Could you check a few things on this model? Use its own coordinates, in mm. Round coordinates to 2 decimals unless told otherwise and drop trailing zeros. Write each loop counter-clockwise with the first axis right and the second up, starting at its lowest first coordinate (ties: lowest second). Pieces come first, ordered by that corner, then holes. Notation, with made-up numbers: (84, -26.5) -> (91, -26.5) arc R13 ccw to (91, -22.5) -> close; hole circle Ø6 at (57.25, 32.5). An arc over 180 degrees is marked (long way). One line per question, with ' | ' between items. Start each with the question number.
1. Thinking about a two-plate mould opening in X: for faces 1 (the cylindrical face through (-98, 2, -99)), 2 (the cylindrical face through (7.509, 1.726, 23.846)), 3 (the cylindrical face through (98, 2, -99)), which applies, released by +X, released by -X, zero draft, split by the parting line, or undercut?
2. Imagine slicing it at B-B, the plane x = 12. List the corners of the cut face in (y, z) for me, and give its area (3 significant figures).
3. Imagine slicing it at A-A, the plane y = 1.8. State how many separate pieces and enclosed holes the cut face has, and give its area (3 significant figures).
4. If I drill on line 1 along X through (y, z) = (2.05, -94); line 2 along Z through (x, y) = (94, 1.75); line 3 along X through (y, z) = (1.9, 90), over which ranges is the centre line in solid material (lowest first)? Write a range as [from, to].
from build123d import *

# Parameters (mm, degrees)
SKETCH_1_R      = 1.55
SKETCH_1_R_2    = 25
SKETCH_1_R_3    = 1.5
EXTRUDE_1_DEPTH = 3.5
FILLET_1_R      = 5


with BuildPart() as part:
    # 草图1 → 凸台-拉伸1 (new body)
    with BuildSketch(Plane(origin=(0, 0, 0), x_dir=(1, 0, 0), z_dir=(0, 1, 0))):
        Polygon((-100, 100), (100, 100), (100, -32.687538375), (100, -80.687538375), (100, -100), (-100, -100), (-100, -80.687538375), (-100, -32.687538375), align=None)
        with Locations(Location((60, 94, 0), (0, 0, 270))):
            Circle(SKETCH_1_R, mode=Mode.SUBTRACT)
        with Locations(Location((60, -94, 0), (0, 0, 270))):
            Circle(SKETCH_1_R, mode=Mode.SUBTRACT)
        with Locations(Location((94, 20, 0), (0, 0, 270))):
            Circle(SKETCH_1_R, mode=Mode.SUBTRACT)
        with Locations(Location((94, -20, 0), (0, 0, 90))):
            Circle(SKETCH_1_R, mode=Mode.SUBTRACT)
        with Locations(Location((-60, -94, 0), (0, 0, 90))):
            Circle(SKETCH_1_R, mode=Mode.SUBTRACT)
        with Locations(Location((-94, -20, 0), (0, 0, 270))):
            Circle(SKETCH_1_R, mode=Mode.SUBTRACT)
        with Locations(Location((-94, 20, 0), (0, 0, 90))):
            Circle(SKETCH_1_R, mode=Mode.SUBTRACT)
        with Locations(Location((-60, 94, 0), (0, 0, 90))):
            Circle(SKETCH_1_R, mode=Mode.SUBTRACT)
        with Locations(Location((0, 0, 0), (0, 0, 270))):
            Circle(SKETCH_1_R_2, mode=Mode.SUBTRACT)
        with Locations(Location((-90, -90, 0), (0, 0, 270))):
            Circle(SKETCH_1_R_3, mode=Mode.SUBTRACT)
        with Locations(Location((-90, 90, 0), (0, 0, 90))):
            Circle(SKETCH_1_R_3, mode=Mode.SUBTRACT)
        with Locations(Location((90, 90, 0), (0, 0, 270))):
            Circle(SKETCH_1_R_3, mode=Mode.SUBTRACT)
        with Locations(Location((90, -90, 0), (0, 0, 90))):
            Circle(SKETCH_1_R_3, mode=Mode.SUBTRACT)
    extrude(amount=EXTRUDE_1_DEPTH)

    # 圆角1
    fillet_1_edges = [part.edges().sort_by_distance(p)[0] for p in [
        (-100, 1.75, -100),
        (100, 1.75, -100),
        (100, 1.75, 100),
        (-100, 1.75, 100),
    ]]
    fillet(fillet_1_edges, radius=FILLET_1_R)


solid = part.part
Geometry results:
1) face 1: released by -X | face 2: undercut | face 3: released by +X
2) outline: (0, -100) -> (3.5, -100) -> (3.5, -21.93) -> (0, -21.93) -> close; (0, 21.93) -> (3.5, 21.93) -> (3.5, 100) -> (0, 100) -> close | area: 546 mm2
3) separate pieces: 1 | enclosed holes: 13 | area: 37,900 mm2
4) line 1: x = [-100, -61.55], [-58.45, 58.45], [61.55, 100] | line 2: z = [-100, -21.55], [-18.45, 18.45], [21.55, 100] | line 3: x = [-100, -91.5], [-88.5, 88.5], [91.5, 100]
